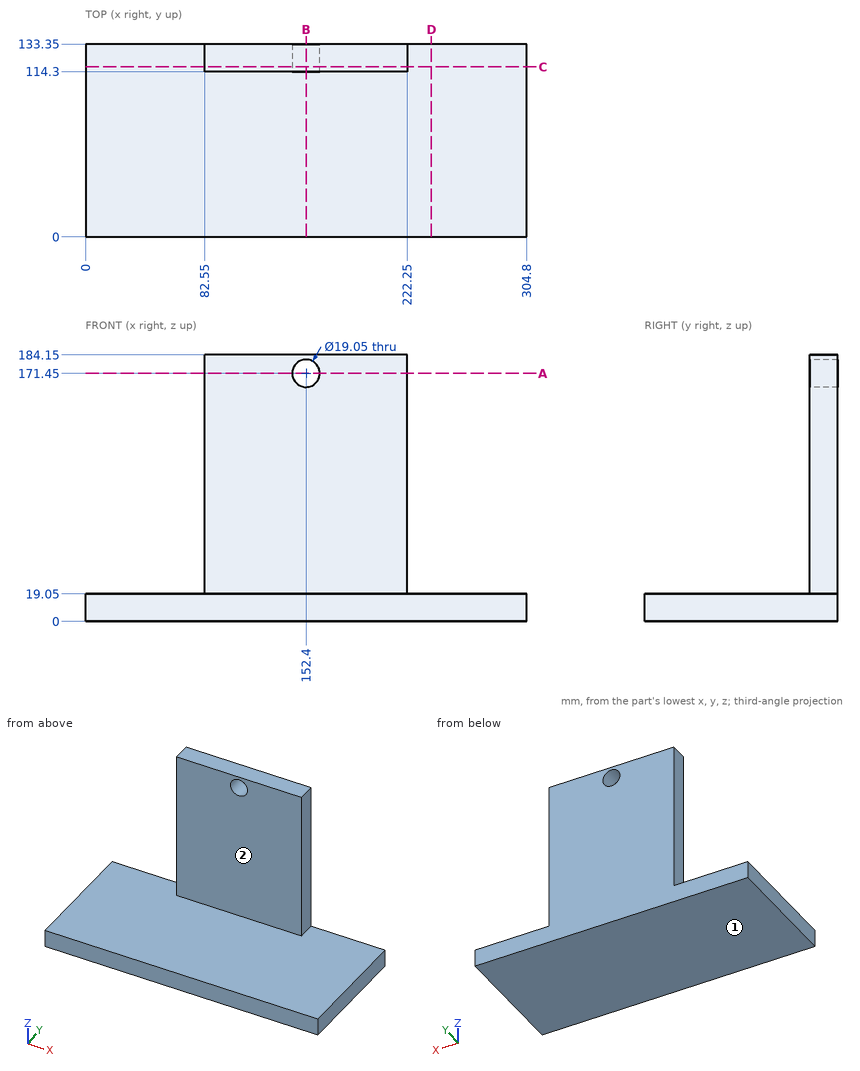
Geometry: see drawing. Coordinates: mm, zero at the bounding-box minimum. A direction names the side the tool comes from. Coordinates: 2 decimals unless noted, no trailing zeros. Write each loop counter-clockwise with the first axis right and the second up, starting at its lowest first coordinate (ties: lowest second). Pieces come first, ordered by that corner, then holes.
1) Material intervals for line 1 along X through (y, z) = (123, 171); line 2 along Z through (x, y) = (152.4, 126.25) (3 decimals); line 3 along Z through (x, y) = (91, 48), sorted ascending.
2) Section D-D on x = 239. Output: boundary loops of the cut face in (y, z), and give its area (3 significant figures).
3) Pin query (flat end, axial travel): pin 1 Ø8 at (x, y) = (265, 59) entering from +Z; pin 2 Ø9.5 at (y, z) = (127, 142) entering from +X; pin 3 Ø21 at (y, z) = (122, 81.5) entering from -X. Return the tip coordinate at first contact, or that it passes through.
4) Section A-A on z = 171.45. Output: boundary loops of the cut face in (x, y) (3 decimals).
5) Section B-B on x = 152.4. Output: boundary loops of the cut face in (y, z) (3 decimals).
6) Set-up query: the marked faces 1 and 2. Return all of +Z, -Z, +X, -X, +Y, -Y with unobstructed straight access to the full face (end or side cutting, diameter ignored); none if empty.
7) Section C-C on y = 117.5. Output: boundary loops of the cut face in (x, z) (3 decimals).
Check result:
1. line 1: x = 82.55 to 142.89, 161.91 to 222.25
1. line 2: z = 0 to 161.925, 180.975 to 184.15
1. line 3: z = 0 to 19.05
2. outline: (0, 0) - (133.35, 0) - (133.35, 19.05) - (0, 19.05) - close
2. area: 2,540 mm2
3. pin 1: stops at z = 19.05
3. pin 2: stops at x = 222.25
3. pin 3: stops at x = 82.55
4. outline: (82.55, 114.3) - (142.875, 114.3) - (142.875, 133.35) - (82.55, 133.35) - close; (161.925, 114.3) - (222.25, 114.3) - (222.25, 133.35) - (161.925, 133.35) - close
5. outline: (0, 0) - (133.35, 0) - (133.35, 161.925) - (114.3, 161.925) - (114.3, 19.05) - (0, 19.05) - close; (114.3, 180.975) - (133.35, 180.975) - (133.35, 184.15) - (114.3, 184.15) - close
6. face 1: -Z, +X, -X, +Y, -Y
6. face 2: +Z, +X, -X, -Y
7. outline: (0, 0) - (304.8, 0) - (304.8, 19.05) - (222.25, 19.05) - (222.25, 184.15) - (82.55, 184.15) - (82.55, 19.05) - (0, 19.05) - close; hole circle Ø19.05 at (152.4, 171.45)
